CAD build for the part. Positions are in the model's coordinates, mm. A direction names the side the tool comes from. Give positions to 0.01 mm unless a question says otherwise; leave off trailing zeros. Loops run counter-clockwise (first coordinate to the right, second up) from the corner with the lowest first, then second, coordinate; pieces in that order, holes last. Notation, with made-up numbers: (82, 43.25) - (96, 43.25) arc R27 cw to (96, 72.25) - close; hole circle Ø10 at (13.25, -39). An arc over 180 degrees is marked (long way). Return JSON: item names as keys, results as strings.
from build123d import *

# Parameters (mm, degrees)
SKETCH1_R           = 9.625
BOSS_EXTRUDE1_DEPTH = 0.625
SKETCH2_R           = 1.225
BOSS_EXTRUDE2_DEPTH = 45
BOSS_EXTRUDE3_DEPTH = 2.4
SKETCH4_R           = 1.25
CUT_EXTRUDE1_DEPTH  = 10


with BuildPart() as part:
    # Sketch1 → Boss-Extrude1 (new, symmetric)
    with BuildSketch(Plane.XY):
        Circle(SKETCH1_R)
    extrude(amount=BOSS_EXTRUDE1_DEPTH, both=True)

    # Sketch2 → Boss-Extrude2 (add)
    with BuildSketch(Plane.XY.offset(0.625)):
        with Locations(Location((0, 0, 0), (0, 0, 180))):
            Circle(SKETCH2_R)
    extrude(amount=BOSS_EXTRUDE2_DEPTH)

    # Sketch3 → Boss-Extrude3 (add, symmetric)
    with BuildSketch(Plane(origin=(0, 0, 0), x_dir=(0, 0, -1), z_dir=(1, 0, 0))):
        with BuildLine():
            Line((-45.625, 5), (-45.625, -5))
            Line((-45.625, -5), (-55.625, -5))
            ThreePointArc((-55.625, -5), (-60.625, 0), (-55.625, 5))
            Line((-55.625, 5), (-45.625, 5))
        make_face()
    extrude(amount=BOSS_EXTRUDE3_DEPTH, both=True)

    # Sketch4 → Cut-Extrude1 (cut)
    with BuildSketch(Plane.ZY.offset(2.4)):
        with Locations((55.625, 0)):
            Circle(SKETCH4_R)
    extrude(amount=-CUT_EXTRUDE1_DEPTH, mode=Mode.SUBTRACT)


solid = part.part
1. Which spindle directions (+Z, -Z, +X, -X, +Y, -Y) get a long thin tool onto all of the face, cutting with end or side? Do faces 4 (the face through (2.4, 0, 53)), 5 (the face through (0, -5, 51)), 6 (the face through (0.9, -0.83, 22.81)). Say none if no direction does.
Values follow:
{"face 4": "+Z, +X, +Y, -Y", "face 5": "+Z, +X, -X, -Y", "face 6": "none"}
2. Cut at B-B, the plane x = 0. Write the cut outline in (y, z) (3 decimals).
Values follow:
{"outline": "(-9.625, -0.625) - (9.625, -0.625) - (9.625, 0.625) - (1.225, 0.625) - (1.225, 45.625) - (5, 45.625) - (5, 55.625) arc R5 ccw to (-5, 55.625) - (-5, 45.625) - (-1.225, 45.625) - (-1.225, 0.625) - (-9.625, 0.625) - close; hole circle Ø2.5 at (0, 55.625)"}
3. Drop flat-ended pins along their axis: P1, Ø4, axis at x = 0, z = 52.5, coming from the -Y side; P2, Ø3, axis at y = 0, z = 54, coming from the -X side; P3, Ø10, axis at y = 3, z = 48, coming from the +X side; P4, Ø8, axis at x = 5.5, z = 6, coming from the +Y side. Give the stop position or say it passes through.
Values follow:
{"P1": "stops at y = -5", "P2": "stops at x = -2.4", "P3": "stops at x = 2.4", "P4": "passes through"}
4. Cut at A-A, the plane y = 0. Write the cut outline in (x, z) (3 decimals).
Values follow:
{"outline": "(-9.625, -0.625) - (9.625, -0.625) - (9.625, 0.625) - (1.225, 0.625) - (1.225, 45.625) - (2.4, 45.625) - (2.4, 54.375) - (-2.4, 54.375) - (-2.4, 45.625) - (-1.225, 45.625) - (-1.225, 0.625) - (-9.625, 0.625) - close; (-2.4, 56.875) - (2.4, 56.875) - (2.4, 60.625) - (-2.4, 60.625) - close"}
5. Cut at D-D, the plane y = -4.25. Write the cut outline in (x, z) (3 decimals).
Values follow:
{"outline": "(-8.636, -0.625) - (8.636, -0.625) - (8.636, 0.625) - (-8.636, 0.625) - close; (-2.4, 45.625) - (2.4, 45.625) - (2.4, 58.259) - (-2.4, 58.259) - close"}
6. Drill centre lines: probe 1 along Z at (x, y) = (2, -3.25) (3 decimals); probe 2 along Z at (x, y) = (1.75, -2.75) (3 decimals); probe 3 along Z at (x, y) = (7, -5) (3 decimals). Where is each one in solid material? Low to high.
Values follow:
{"probe 1": "z = -0.625 to 0.625, 45.625 to 59.425", "probe 2": "z = -0.625 to 0.625, 45.625 to 59.801", "probe 3": "z = -0.625 to 0.625"}
7. Pull direction Y, two halves, no side cores. Call faces 1 (the face through (1, 1, 45.625)), 2 (the face through (-0.034, 0.375, 56.817)), 3 (the face through (0, 5, 51)): +Y half, -Y half, draft (parallel to the pull), parting line (faces both ways), or undercut.
Values follow:
{"face 1": "draft", "face 2": "undercut", "face 3": "+Y half"}
8. Cut at C-C, the plane z = 26.5. Write the cut outline in (x, y) (3 decimals), plus the area to 3 significant figures.
Values follow:
{"outline": "circle Ø2.45 at (0, 0)", "area": "4.71 mm²"}
